Geometry check sheet. Reference: the model listing, model coordinates, mm. Face numbers are marked on the shaded views. A direction names the side the tool comes from. Round coordinates to 2 decimals unless told otherwise and drop trailing zeros. Order: outer loops, then holes, each group sorted by start corner. A loop starts at its lowest first (then second) coordinate and runs counter-clockwise, first axis right, second up. Notation, with made-up numbers: (15.25, -30) - (19.25, -30) arc R14 ccw to (19.25, -23) - close; hole circle Ø7 at (68.5, -34.5). An arc over 180 degrees is marked (long way). Use a Markdown table: item, result. Add a question column.
(1) Access from +Z, -Z, +X, -X, +Y, -Y to the whole of each face (thin tool, end or side, straight path). Record for the marked faces 1, 2, 3, 4 and 5.
(2) Section check D-D on x = 0. Record the boundary of the cut face in (y, z), then the cut area to 3 significant figures.
(3) Thickness scan on line 1 along Y through (x, z) = (-34.5, 0); line 2 along X through (y, z) = (5, -1); line 3 along Z through (x, y) = (-33.25, 0). Record the ranges inside material, lowest first. Write a range as [from, to].
(4) Section check C-C on z = 23. Record the boundary of the cut face in (x, y).
(5) Section check A-A on z = 0. Record the boundary of the cut face in (x, y), then the cut area to 3 significant figures.
(6) Gauge pin test, flat ends, axial feed: P1, Ø2, axis at y = 5, z = 10, coming from the -X side; P2, Ø1.5, axis at x = -27.5, y = -2, coming from the -Z side; P3, Ø5, axis at x = 36, y = 2.5, coming from the +Z side. Record the tip position at first contact, or that the pin passes through.
(7) Section check B-B on x = 34. Record the boundary of the cut face in (y, z).
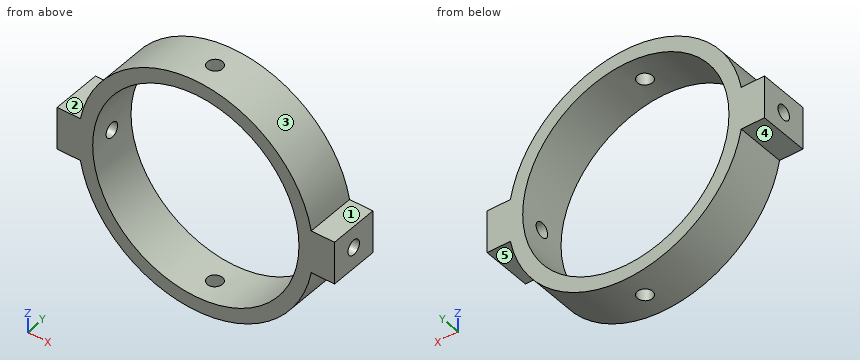
```python
from build123d import *

# Parameters (mm, degrees)
SKETCH1_R               = 33
SKETCH1_R_2             = 29
BOSS_EXTRUDE1_DEPTH     = 7
SKETCH2_W               = 10
SKETCH2_H               = 12
BOSS_EXTRUDE2_DEPTH     = 7
SKETCH5_R               = 2.1
CUT_EXTRUDE1_DEPTH      = 85.982351109
CUT_EXTRUDE4_DEPTH      = 52.565492427
CUT_EXTRUDE4_DEPTH_BACK = 52.565492427
SKETCH7_R               = 2.1


with BuildPart() as part:
    # Sketch1 → Boss-Extrude1 (new, symmetric)
    with BuildSketch(Plane(origin=(0, 0, 0), x_dir=(1, 0, 0), z_dir=(0, 1, 0))):
        with Locations(Location((0, 0, 0), (0, 0, 270))):
            Circle(SKETCH1_R)
        with Locations(Location((0, 0, 0), (0, 0, 270))):
            Circle(SKETCH1_R_2, mode=Mode.SUBTRACT)
    extrude(amount=BOSS_EXTRUDE1_DEPTH, both=True)

    # Sketch2 → Boss-Extrude2 (add, symmetric)
    with BuildSketch(Plane(origin=(0, 0, 0), x_dir=(1, 0, 0), z_dir=(0, 1, 0))):
        with Locations((34, 0)):
            Rectangle(SKETCH2_W, SKETCH2_H)
        with Locations((-34, 0)):
            Rectangle(SKETCH2_W, SKETCH2_H)
    extrude(amount=BOSS_EXTRUDE2_DEPTH, both=True)

    # Sketch5 → Cut-Extrude1 (cut, through all)
    with BuildSketch(Plane.ZY.offset(39)):
        Circle(SKETCH5_R)
    extrude(amount=-CUT_EXTRUDE1_DEPTH, mode=Mode.SUBTRACT)

    # Sketch7 → Cut-Extrude4 (cut, two sides: drawn at the far end of the back side and taken through both)
    with BuildSketch(Plane.XY.offset(-CUT_EXTRUDE4_DEPTH_BACK)):
        Circle(SKETCH7_R)
    extrude(amount=CUT_EXTRUDE4_DEPTH + CUT_EXTRUDE4_DEPTH_BACK, mode=Mode.SUBTRACT)


solid = part.part
```
Check sheet entries:
| question | item | result |
|---|---|---|
| 1 | face 1 | +Z, +X, +Y, -Y |
| 1 | face 2 | +Z, -X, +Y, -Y |
| 1 | face 3 | +Z, +Y, -Y |
| 1 | face 4 | -Z, -X, +Y, -Y |
| 1 | face 5 | -Z, +X, +Y, -Y |
| 2 | outline | (-7, -33) - (-2.1, -33) - (-2.1, -29) - (-7, -29) - close; (-7, 29) - (-2.1, 29) - (-2.1, 33) - (-7, 33) - close; (2.1, -33) - (7, -33) - (7, -29) - (2.1, -29) - close; (2.1, 29) - (7, 29) - (7, 33) - (2.1, 33) - close |
| 2 | area | 78.4 mm2 |
| 3 | line 1 | y = [-7, -2.1], [2.1, 7] |
| 3 | line 2 | x = [-39, -28.98], [28.98, 39] |
| 3 | line 3 | z = [-6, -2.1], [2.1, 6] |
| 4 | outline | (-23.66, -7) - (-17.66, -7) - (-17.66, 7) - (-23.66, 7) - close; (17.66, -7) - (23.66, -7) - (23.66, 7) - (17.66, 7) - close |
| 5 | outline | (-39, -7) - (-29, -7) - (-29, -2.1) - (-39, -2.1) - close; (-39, 2.1) - (-29, 2.1) - (-29, 7) - (-39, 7) - close; (29, -7) - (39, -7) - (39, -2.1) - (29, -2.1) - close; (29, 2.1) - (39, 2.1) - (39, 7) - (29, 7) - close |
| 5 | area | 196 mm2 |
| 6 | P1 | stops at x = -31.75 |
| 6 | P2 | stops at z = -19.32 |
| 6 | P3 | stops at z = 6 |
| 7 | outline | (-7, -6) - (7, -6) - (7, 6) - (-7, 6) - close; hole circle Ø4.2 at (0, 0) |
